Part model, mm, in its own coordinate system. Give positions to 0.01 mm unless a question says otherwise; leave off trailing zeros. Order: outer loops, then holes, each group sorted by start corner. A loop starts at its lowest first (then second) coordinate and runs counter-clockwise, first axis right, second up. Notation, with made-up numbers: (43, 20.5) - (70, 20.5) arc R22 cw to (70, 55.5) - close; hole circle Ø4 at (65.5, 15.25). An arc over 180 degrees is marked (long way). One line per item, written item: value.
```python
from build123d import *

# Parameters (mm, degrees)
EXTRUDE_THIN1_DEPTH = 1524
FILLET1_R           = 1.27


with BuildPart() as part:
    # Sketch1 → Extrude-Thin1 (new body)
    with BuildSketch(Plane.XY):
        with BuildLine():
            Line((0, 6.858), (0, 0))
            Line((0, 0), (-12.7, 0))
            Line((-12.7, 0), (-12.7, 142.875))
            ThreePointArc((-12.7, 142.875), (-8.674261314, 150.652129933), (0, 151.855256121))
            Line((0, 151.855256121), (0, 144.997256121))
            Line((0, 144.997256121), (-1.27, 144.997256121))
            Line((-1.27, 144.997256121), (-1.27, 150.907185257))
            ThreePointArc((-1.27, 150.907185257), (-8.29453367, 149.350754782), (-11.43, 142.875))
            Line((-11.43, 142.875), (-11.43, 1.27))
            Line((-11.43, 1.27), (-1.27, 1.27))
            Line((-1.27, 1.27), (-1.27, 6.858))
            Line((-1.27, 6.858), (0, 6.858))
        make_face()
    extrude(amount=-EXTRUDE_THIN1_DEPTH)

    # Fillet1
    fillet1_edges = [part.edges().sort_by_distance(p)[0] for p in [
        (0, 0, -762),
        (-12.7, 0, -762),
        (0, 151.855256121, -762),
    ]]
    fillet(fillet1_edges, radius=FILLET1_R)


solid = part.part
```
1) Drill centre lines: line 1 along Y through (x, z) = (-2, -353.5); line 2 along Y through (x, z) = (-5.25, -68); line 3 along X through (y, z) = (51.5, -391). Where is each one in solid material? Low to high. Write a range as from..to.
Outcome:
line 1: y = 0..1.27, 151.05..152.33
line 2: y = 0..1.27, 150.86..152.17
line 3: x = -12.7..-11.43
2) Cut at A-A, the plane z = -1198.5. Give the cut face in (x, y) (3 decimals), then the cut area to 3 significant figures.
Outcome:
outline: (-12.7, 1.27) arc R1.27 ccw to (-11.43, 0) - (-1.27, 0) arc R1.27 ccw to (0, 1.27) - (0, 6.858) - (-1.27, 6.858) - (-1.27, 1.27) - (-11.43, 1.27) - (-11.43, 142.875) arc R8.255 cw to (-1.27, 150.907) - (-1.27, 144.997) - (0, 144.997) - (0, 150.907) arc R1.27 ccw to (-0.977, 152.143) arc R9.525 ccw to (-12.7, 142.875) - close
area: 231 mm^2
3) Mould opens along Y. For faces 1 (the flat face through (-12.7, 71, -751)), 2 (the flat face through (-11.43, 73, -751)) say: released by +Y, released by -Y, zero draft, split by the parting line, or undercut.
Outcome:
face 1: zero draft
face 2: undercut
4) Pin check, flat tips, straight feed: pin 1 (3 mm diameter, centred on y = 78, z = -156, fed in from +X); pin 2 (0.6 mm diameter, centred on x = -0.5, z = -720, fed in from -Y); pin 3 (1 mm diameter, centred on x = -0.5, z = -575.5, fed in from +Y). Stop position of each tip, or through.
Outcome:
pin 1: stops at x = -11.43
pin 2: stops at y = 0.09
pin 3: stops at y = 152.15
5) Cut at B-B, the plane x = -4.75. Give the cut face in (y, z), then the cut area to 3 significant figures.
Outcome:
outline: (0, -1524) - (1.27, -1524) - (1.27, 0) - (0, 0) - close; (150.98, -1524) - (152.27, -1524) - (152.27, 0) - (150.98, 0) - close
area: 3,900 mm^2
6) Cut at C-C, the plane y = 113. Give the cut face in (x, z).
Outcome:
outline: (-12.7, -1524) - (-11.43, -1524) - (-11.43, 0) - (-12.7, 0) - close
